from build123d import *

# Parameters (mm, degrees)
SKETCH_1_R          = 7.5
EXTRUDE_1_DEPTH     = 4
SKETCH_4_R          = 1
CUT_EXTRUDE_2_DEPTH = 4


with BuildPart() as part:
    # Эскиз1 → Бобышка-Вытянуть1 (new body)
    with BuildSketch(Plane.XY):
        Circle(SKETCH_1_R)
    extrude(amount=EXTRUDE_1_DEPTH)

    # Эскиз4 → Вырез-Вытянуть2 (cut)
    with BuildSketch(Plane.XY.offset(4)):
        with Locations((0, 5.25)):
            Circle(SKETCH_4_R)
        with Locations((0, -5.25)):
            Circle(SKETCH_4_R)
        with BuildLine():
            Line((-1.58113883, 2.25), (1.58113883, 2.25))
            ThreePointArc((1.58113883, 2.25), (2.75, 0), (1.58113883, -2.25))
            Line((1.58113883, -2.25), (-1.58113883, -2.25))
            ThreePointArc((-1.58113883, -2.25), (-2.75, 0), (-1.58113883, 2.25))
        make_face()
    extrude(amount=-CUT_EXTRUDE_2_DEPTH, mode=Mode.SUBTRACT)


solid = part.part
Verification items for the finished model (mm, model axes). A direction names the side the tool comes from. Give positions to 0.01 mm unless a question says otherwise; leave off trailing zeros. Order: outer loops, then holes, each group sorted by start corner. A loop starts at its lowest first (then second) coordinate and runs counter-clockwise, first axis right, second up. Notation, with made-up numbers: M -9,50.5 L 0,50.5 A19 ccw 0,54.5 Z; hole C 4,81.5 d6. An arc over 180 degrees is marked long. Answer as a JSON object with one key per item and string values. Group by question number.
1) Mould release check, pull along Y, two halves, no side actions. Record for faces 1 (the face through (-0.13, -4.26, 2.03)), 2 (the face through (3, 0, 0)), 3 (the face through (-7.493, 0.33, 1.972)): released by +Y, released by -Y, zero draft, split by the parting line, or undercut.
2) Cross-section at A-A (x = 0). Enter the section's corners in (y, z), then the cut area to 3 significant figures.
3) Access from +Z, -Z, +X, -X, +Y, -Y to the whole of each face (thin tool, end or side, straight path). Record for faces 4 (the face through (0, -2.25, 2)), 5 (the face through (3, 0, 4)).
4) Cross-section at C-C (z = 0.85). Enter the section's corners in (x, y).
5) Scan lines: line 1 along Y through (x, z) = (0, 1); line 2 along Y through (x, z) = (-1.5, 1.4); line 3 along X through (y, z) = (-6, 0.25). Record each from-to range of solid material in increasing order. Write a range as [from, to].
6) Cross-section at B-B (y = -6). Enter the section's corners in (x, z), then the cut area to 3 significant figures.
7) Cross-section at D-D (x = -2.5). Enter the section's corners in (y, z), then the cut area to 3 significant figures.
8) Depth check by flat-ended pin: pin 1 Ø4 at (x, y) = (0, -0.5) entering from -Z; pin 2 Ø1.5 at (x, z) = (-6, 1) entering from +Y. Enter the tip coordinate at first touch or a pass-through.
Result sheet:
{
 "1": {"face 1": "undercut", "face 2": "zero draft", "face 3": "split by the parting line"},
 "2": {"outline": "M -7.5,0 L -6.25,0 L -6.25,4 L -7.5,4 Z; M -4.25,0 L -2.25,0 L -2.25,4 L -4.25,4 Z; M 2.25,0 L 4.25,0 L 4.25,4 L 2.25,4 Z; M 6.25,0 L 7.5,0 L 7.5,4 L 6.25,4 Z", "area": "26.0 mm2"},
 "3": {"face 4": "+Z, -Z", "face 5": "+Z, +X, -X, +Y, -Y"},
 "4": {"outline": "C 0,0 d15; hole M -1.58,-2.25 L 1.58,-2.25 A2.75 ccw 1.58,2.25 L -1.58,2.25 A2.75 ccw Z; hole C 0,-5.25 d2; hole C 0,5.25 d2"},
 "5": {"line 1": "y = [-7.5, -6.25], [-4.25, -2.25], [2.25, 4.25], [6.25, 7.5]", "line 2": "y = [-7.35, -2.25], [2.25, 7.35]", "line 3": "x = [-4.5, -0.66], [0.66, 4.5]"},
 "6": {"outline": "M -4.5,0 L -0.66,0 L -0.66,4 L -4.5,4 Z; M 0.66,0 L 4.5,0 L 4.5,4 L 0.66,4 Z", "area": "30.7 mm2"},
 "7": {"outline": "M -7.07,0 L -1.15,0 L -1.15,4 L -7.07,4 Z; M 1.15,0 L 7.07,0 L 7.07,4 L 1.15,4 Z", "area": "47.4 mm2"},
 "8": {"pin 1": "stops at z = 0", "pin 2": "stops at y = 5.36"}
}
